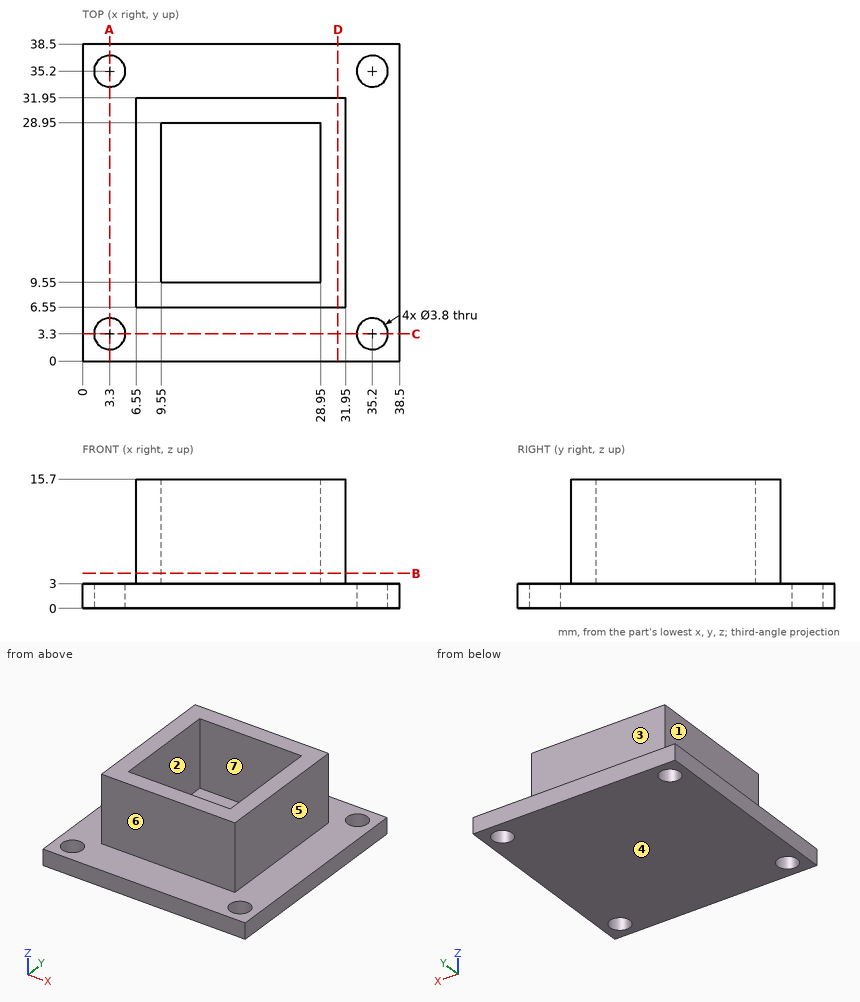
Geometry check sheet. Reference: drawing and pictorial views, mm from the part's lowest x, y, z. A direction names the side the tool comes from. Round coordinates to 2 decimals unless told otherwise and drop trailing zeros. Order: outer loops, then holes, each group sorted by start corner. A loop starts at its lowest first (then second) coordinate and runs counter-clockwise, first axis right, second up. Notation, with made-up numbers: M 20.25,-34 L 68.25,-34 A20 cw 68.25,-13 Z; hole C 31.5,6.25 d7. An arc over 180 degrees is marked long. Answer as CSV lines item,"result".
1) Tool access check on the marked faces 1, 2, 3 and 4. Record the directions out of +Z, -Z, +X, -X, +Y, -Y that give a thin tool (end or side, any length) a straight path to the whole face; none if there is none.
Entries:
face 1,"+Z, -X, +Y, -Y"
face 2,"+Z"
face 3,"+Z, +X, -X, +Y"
face 4,"-Z, +X, -X, +Y, -Y"
2) Gauge pin test, flat ends, axial feed: pin 1 Ø6.5 at (y, z) = (18, 9) entering from +X; pin 2 Ø3 at (y, z) = (20.5, 6) entering from -X; pin 3 Ø4.5 at (x, y) = (35.2, 3.3) entering from +Z. Record the tip position at first contact, or that the pin passes through.
Entries:
pin 1,"x = 31.95"
pin 2,"x = 6.55"
pin 3,"z = 3"
3) Sectioned sample at A-A on x = 3.3. Record the cut outline in (y, z).
Entries:
outline,"M 0,0 L 1.4,0 L 1.4,3 L 0,3 Z; M 5.2,0 L 33.3,0 L 33.3,3 L 5.2,3 Z; M 37.1,0 L 38.5,0 L 38.5,3 L 37.1,3 Z"
4) Sectioned sample at B-B on z = 4.25. Record the cut outline in (x, y).
Entries:
outline,"M 6.55,6.55 L 31.95,6.55 L 31.95,31.95 L 6.55,31.95 Z; hole M 9.55,9.55 L 28.95,9.55 L 28.95,28.95 L 9.55,28.95 Z"
5) Sectioned sample at D-D on x = 31. Record the cut outline in (y, z).
Entries:
outline,"M 0,0 L 38.5,0 L 38.5,3 L 31.95,3 L 31.95,15.7 L 6.55,15.7 L 6.55,3 L 0,3 Z"
6) Thickness scan on probe 1 along X at (y, z) = (35.2, 0.85); probe 2 along X at (y, z) = (12, 7.25). Record the ranges inside material, lowest first. Write a range as [from, to].
Entries:
probe 1,"[0, 1.4], [5.2, 33.3], [37.1, 38.5]"
probe 2,"[6.55, 9.55], [28.95, 31.95]"
7) Mould release check, pull along Y, two halves, no side actions. Record for the marked faces 5, 6 and 7: +Y half, -Y half, draft (parallel to the pull), parting line (faces both ways), or undercut.
Entries:
face 5,"draft"
face 6,"-Y half"
face 7,"undercut"
